```python
from build123d import *

# Parameters (mm, degrees)
SKETCH1_R           = 6.011
SKETCH1_W           = 6.016
SKETCH1_H           = 6.016
BOSS_EXTRUDE1_DEPTH = 5.5
BOSS_EXTRUDE2_START = 2
SKETCH1_3_R         = 8
SKETCH1_3_R_2       = 6.011
SKETCH1_3_W         = 6.016
SKETCH1_3_H         = 6.016
BOSS_EXTRUDE2_DEPTH = 2
FILLET1_R           = 0.5
CUT_EXTRUDE1_DEPTH  = 0.5


with BuildPart() as part:
    # Sketch1 → Boss-Extrude1 (new body)
    with BuildSketch(Plane.XY):
        Circle(SKETCH1_R)
        Rectangle(SKETCH1_W, SKETCH1_H, mode=Mode.SUBTRACT)
    extrude(amount=-BOSS_EXTRUDE1_DEPTH)

    # Sketch1_3 → Boss-Extrude2 (add)
    # profile 1 of 2: a face of its own
    with BuildSketch(Plane.XY.offset(BOSS_EXTRUDE2_START)):
        Circle(SKETCH1_3_R)
        Circle(SKETCH1_3_R_2, mode=Mode.SUBTRACT)
    # profile 2 of 2: a face of its own
    with BuildSketch(Plane.XY.offset(BOSS_EXTRUDE2_START)):
        Circle(SKETCH1_3_R_2)
        Rectangle(SKETCH1_3_W, SKETCH1_3_H, mode=Mode.SUBTRACT)
    extrude(amount=-BOSS_EXTRUDE2_DEPTH)

    # Fillet1
    fillet1_edges = [part.edges().sort_by_distance(p)[0] for p in [
        (-8, 0, 0),
        (-6.011, 0, -5.5),
    ]]
    fillet(fillet1_edges, radius=FILLET1_R)

    # Sketch2 → Cut-Extrude1 (cut)
    with BuildSketch(Plane.XY.offset(2)):
        with BuildLine():
            Line((-0.770976701, 6.337168177), (-1.085079266, 6.337168177))
            add(Edge.make_bspline(
                [(-1.085079266, 6.337168177), (-1.076569715, 6.372400661), (-1.059934239, 6.441277286), (-1.025236666, 6.539684546), (-0.987437411, 6.632808068), (-0.942048306, 6.718904141), (-0.892539552, 6.799703044), (-0.83581683, 6.873372169), (-0.774497108, 6.941785134), (-0.706672158, 7.002498372), (-0.635543497, 7.057476101), (-0.560108877, 7.104351158), (-0.481885983, 7.144675311), (-0.40033285, 7.177895543), (-0.315206679, 7.202921067), (-0.227277055, 7.221077872), (-0.136313555, 7.232868986), (-0.074565965, 7.23401975), (-0.043212278, 7.234604075)],
                knots=[0, 0, 0, 0, 1.162005537, 2.271625781, 3.343758855, 4.383309926, 5.390229558, 6.379919256, 7.361854164, 8.333198761, 9.295911338, 10.242430842, 11.177959212, 12.116337295, 13.062827104, 14.020064771, 14.994644689, 16, 16, 16, 16], degree=3))
            add(Edge.make_bspline(
                [(-0.043212278, 7.234604075), (0.002470464, 7.233224844), (0.092839475, 7.230496469), (0.225602522, 7.205582032), (0.353629341, 7.1661569), (0.475518589, 7.111683173), (0.588737021, 7.04449586), (0.689473208, 6.964531123), (0.776361719, 6.873331821), (0.849256096, 6.772599257), (0.906331095, 6.664943748), (0.948417469, 6.554143591), (0.97403915, 6.440461619), (0.977359707, 6.36370434), (0.979023299, 6.325249107)],
                knots=[0, 0, 0, 0, 1.083050992, 2.142477498, 3.193116406, 4.255571735, 5.30263384, 6.308962982, 7.297363603, 8.282367274, 9.249857812, 10.179914175, 11.08814088, 12, 12, 12, 12], degree=3))
            add(Edge.make_bspline(
                [(0.979023299, 6.325249107), (0.977859708, 6.288242312), (0.97558274, 6.215825757), (0.956249035, 6.11010426), (0.923712772, 6.01046266), (0.878643009, 5.916481498), (0.820301459, 5.828756658), (0.749628762, 5.747090767), (0.6661261, 5.671121609), (0.602847162, 5.627602136), (0.570269292, 5.605197023)],
                knots=[0, 0, 0, 0, 1.024540389, 2.004866551, 2.965041327, 3.920577974, 4.882998113, 5.874504559, 6.905732034, 8, 8, 8, 8], degree=3))
            add(Edge.make_bspline(
                [(0.570269292, 5.605197023), (0.607501047, 5.587218852), (0.681267921, 5.551598894), (0.781818451, 5.481743137), (0.873096326, 5.401086789), (0.924000045, 5.338144136), (0.949576183, 5.306519139)],
                knots=[0, 0, 0, 0, 1.015518401, 2.012035669, 3.001164323, 4, 4, 4, 4], degree=3))
            add(Edge.make_bspline(
                [(0.949576183, 5.306519139), (0.966417526, 5.283461387), (0.999824422, 5.237723471), (1.041059955, 5.164187045), (1.07846907, 5.089835555), (1.107619289, 5.012676149), (1.130193156, 4.933603136), (1.146329188, 4.85248074), (1.156353329, 4.769242717), (1.157788881, 4.712930237), (1.158510478, 4.684624107)],
                knots=[0, 0, 0, 0, 1.025084078, 2.033381695, 3.024893161, 4.013698104, 4.991890475, 5.976764909, 6.982997093, 8, 8, 8, 8], degree=3))
            add(Edge.make_bspline(
                [(1.158510478, 4.684624107), (1.156715965, 4.635614385), (1.153135383, 4.537825584), (1.121131308, 4.393350862), (1.071518068, 4.25212536), (1.001061132, 4.11705052), (0.915193623, 3.990670139), (0.813036299, 3.87759383), (0.69574989, 3.780395226), (0.564944241, 3.699184998), (0.423227113, 3.634267076), (0.271651521, 3.589209633), (0.112401467, 3.559863633), (0.003194169, 3.556716764), (-0.052326862, 3.555116895)],
                knots=[0, 0, 0, 0, 0.955779014, 1.907060117, 2.875433937, 3.871313158, 4.872415639, 5.851225146, 6.836215519, 7.83643374, 8.849228613, 9.86973379, 10.916971861, 12, 12, 12, 12], degree=3))
            add(Edge.make_bspline(
                [(-0.052326862, 3.555116895), (-0.089746162, 3.555985108), (-0.163374867, 3.557693463), (-0.271618365, 3.569372064), (-0.374940065, 3.590702069), (-0.473479663, 3.619405374), (-0.567324699, 3.655797116), (-0.656188804, 3.701115814), (-0.740618698, 3.754427316), (-0.819817649, 3.816360904), (-0.893776217, 3.885642244), (-0.960528941, 3.963501254), (-1.021188734, 4.048498658), (-1.074131372, 4.141621714), (-1.121768325, 4.241666971), (-1.160949282, 4.34991547), (-1.19543485, 4.465399492), (-1.211468315, 4.545877232), (-1.21969465, 4.587168177)],
                knots=[0, 0, 0, 0, 1.048658725, 2.063410685, 3.046034179, 4.001477787, 4.936774919, 5.862367409, 6.792675028, 7.730719943, 8.675894397, 9.627829632, 10.600096036, 11.597688215, 12.626045268, 13.701542398, 14.82072376, 16, 16, 16, 16], degree=3))
            Line((-1.21969465, 4.587168177), (-0.905592086, 4.587168177))
            add(Edge.make_bspline(
                [(-0.905592086, 4.587168177), (-0.897408795, 4.560219164), (-0.881491582, 4.507800992), (-0.854397284, 4.432360687), (-0.823529012, 4.363202633), (-0.790414453, 4.299819511), (-0.755636007, 4.241587109), (-0.716721082, 4.19004524), (-0.676551937, 4.142930038), (-0.646272584, 4.116385426), (-0.631453464, 4.103394139)],
                knots=[0, 0, 0, 0, 1.198163088, 2.33053128, 3.407730985, 4.417276592, 5.372219308, 6.28897303, 7.162600585, 8, 8, 8, 8], degree=3))
            add(Edge.make_bspline(
                [(-0.631453464, 4.103394139), (-0.611856888, 4.088285805), (-0.572724225, 4.058115773), (-0.508955994, 4.019614144), (-0.441891108, 3.986253119), (-0.370076433, 3.960769423), (-0.295061663, 3.939191763), (-0.215634298, 3.925071244), (-0.132495081, 3.915383072), (-0.075727317, 3.914528141), (-0.046717887, 3.914091254)],
                knots=[0, 0, 0, 0, 0.946170439, 1.889420265, 2.845303464, 3.807233317, 4.801018734, 5.828864929, 6.890507805, 8, 8, 8, 8], degree=3))
            add(Edge.make_bspline(
                [(-0.046717887, 3.914091254), (-0.013964385, 3.914707159), (0.050082262, 3.915911509), (0.143537122, 3.926987216), (0.232444569, 3.943117629), (0.315817495, 3.968030612), (0.394748002, 3.998811463), (0.468129652, 4.037459869), (0.536925758, 4.082804591), (0.600255164, 4.134343749), (0.657200671, 4.190765244), (0.707340184, 4.249778315), (0.749964846, 4.311134145), (0.784348424, 4.375172266), (0.811498974, 4.441627495), (0.829982175, 4.510686324), (0.84283369, 4.58178359), (0.843880302, 4.630112559), (0.844407914, 4.654475869)],
                knots=[0, 0, 0, 0, 1.217147791, 2.380027433, 3.494444702, 4.572153297, 5.609568379, 6.639424714, 7.649109417, 8.668170816, 9.669597737, 10.625200337, 11.543417969, 12.441394052, 13.322311151, 14.205496177, 15.095365482, 16, 16, 16, 16], degree=3))
            add(Edge.make_bspline(
                [(0.844407914, 4.654475869), (0.842877612, 4.687087208), (0.839824624, 4.752147617), (0.816516045, 4.847865191), (0.77817718, 4.940088603), (0.724504669, 5.027244393), (0.65916894, 5.108020295), (0.582804033, 5.180091777), (0.494775805, 5.239561868), (0.413755936, 5.280650525), (0.34199078, 5.3086876), (0.280575395, 5.327362564), (0.211818792, 5.34317622), (0.136552443, 5.357888492), (0.054209226, 5.37040984), (-0.035121212, 5.380851656), (-0.131456973, 5.389206697), (-0.198148139, 5.392937792), (-0.232515163, 5.394860485)],
                knots=[0, 0, 0, 0, 1.07054697, 2.135767047, 3.216561865, 4.33974944, 5.486079747, 6.621378074, 7.775625952, 8.963672916, 9.598146892, 10.304877434, 11.070270905, 11.915000392, 12.823868403, 13.805723172, 14.86925407, 16, 16, 16, 16], degree=3))
            Line((-0.232515163, 5.394860485), (-0.232515163, 5.753834844))
            add(Edge.make_bspline(
                [(-0.232515163, 5.753834844), (-0.189213997, 5.754569648), (-0.104397651, 5.756008948), (0.019496654, 5.773416958), (0.137969966, 5.797497586), (0.248396708, 5.834382778), (0.349045422, 5.877223075), (0.436365024, 5.927075285), (0.509132171, 5.982490034), (0.566993242, 6.044322643), (0.610522471, 6.110637691), (0.642349268, 6.179754348), (0.661149595, 6.252278409), (0.663659262, 6.301773077), (0.664920734, 6.32665135)],
                knots=[0, 0, 0, 0, 1.321986639, 2.589447074, 3.816329219, 5.01088745, 6.139805852, 7.153945165, 8.075214402, 8.924034688, 9.728124013, 10.488707548, 11.240355623, 12, 12, 12, 12], degree=3))
            add(Edge.make_bspline(
                [(0.664920734, 6.32665135), (0.664506324, 6.344929095), (0.663681873, 6.381291802), (0.653284595, 6.434416871), (0.637660554, 6.485917817), (0.616180824, 6.535575627), (0.587430626, 6.583045901), (0.553024639, 6.62873335), (0.512056539, 6.672377129), (0.465111092, 6.713057449), (0.414699287, 6.751826686), (0.359449512, 6.784740323), (0.301027637, 6.812885385), (0.239368982, 6.836094887), (0.174273452, 6.853554175), (0.106046894, 6.866090017), (0.034559211, 6.873927671), (-0.014212521, 6.875056087), (-0.039005548, 6.875629716)],
                knots=[0, 0, 0, 0, 0.884392785, 1.759457502, 2.611959086, 3.489218968, 4.37281399, 5.2945488, 6.255912374, 7.266815255, 8.301784654, 9.332968512, 10.37626691, 11.440494194, 12.520033166, 13.637162961, 14.798855837, 16, 16, 16, 16], degree=3))
            add(Edge.make_bspline(
                [(-0.039005548, 6.875629716), (-0.078857216, 6.874238354), (-0.156696792, 6.8715207), (-0.268911709, 6.847717687), (-0.373231043, 6.809739603), (-0.452969709, 6.764406584), (-0.511852284, 6.71965615), (-0.553929222, 6.680573763), (-0.595249732, 6.63714094), (-0.633095409, 6.586682564), (-0.671369386, 6.532615774), (-0.706213947, 6.472192093), (-0.74007364, 6.406987698), (-0.760476189, 6.360892064), (-0.770976701, 6.337168177)],
                knots=[0, 0, 0, 0, 1.472543308, 2.876219568, 4.221790263, 5.565193594, 6.249813518, 6.953379497, 7.687249741, 8.463570142, 9.283606569, 10.136032583, 11.040678096, 12, 12, 12, 12], degree=3))
        make_face()
    extrude(amount=-CUT_EXTRUDE1_DEPTH, mode=Mode.SUBTRACT)


solid = part.part
```
Geometry check sheet. Reference: the model listing, model coordinates, mm. A direction names the side the tool comes from. Coordinates: 2 decimals unless noted, no trailing zeros. Loops run counter-clockwise (first coordinate to the right, second up) from the corner with the lowest first, then second, coordinate; pieces in that order, holes last. Notation, with made-up numbers: (18, 50) - (25, 50) arc R29 cw to (25, 76) - close; hole circle Ø1 at (60, 16). An arc over 180 degrees is marked (long way). One line per item, written item: value. Start each with the question number.
(1) Mould release check, pull along Y, two halves, no side actions. Record for faces 5 (the flat face through (0, 3.008, -2)), 6 (the flat face through (-6, 2, 0)), 7 (the cylindrical face through (-1.73, -7.81, 1.26)): released by +Y, released by -Y, zero draft, split by the parting line, or undercut.
(2) Material ranges on line 1 (X direction, y = 0.25, z = 1.25); line 2 (Z direction, x = 6.25, y = -2.25); line 3 (X direction, y = -0.5, z = -3.75), recorded low to high. Write a range as [from, to].
(3) Cross-section at B-B on z = -3.5. Enter the section's corners in (x, y).
(4) Tool access check on faces 1 (the cylindrical face through (-0.78, 5.96, -2.46)), 2 (the flat face through (0.06, 5.54, 1.5)), 3 (the flat face through (-3.008, 0, -2)), 4 (the flat face through (0, -4, -5.5)). Record the directions out of +Z, -Z, +X, -X, +Y, -Y that give a thin tool (end or side, any length) a straight path to the whole face; none if there is none.
(5) Depth check by flat-ended pin: P1, Ø1.5, axis at y = 1, z = 0, coming from the -X side; P2, Ø3, axis at x = 1, z = -3, coming from the -Y side; P3, Ø1, axis at y = -2, z = -4, coming from the +X side. Enter the tip coordinate at first touch or a pass-through.
(6) Cross-section at A-A on y = 0. Enter the section's corners in (x, z), plus the area to 3 significant figures.
Results below:
1. face 5: undercut
1. face 6: zero draft
1. face 7: split by the parting line
2. line 1: x = [-8, -3.01], [3.01, 8]
2. line 2: z = [0, 2]
2. line 3: x = [-5.99, -3.01], [3.01, 5.99]
3. outline: circle Ø12.02 at (0, 0); hole (-3.01, -3.01) - (3.01, -3.01) - (3.01, 3.01) - (-3.01, 3.01) - close
4. face 1: -Z
4. face 2: +Z
4. face 3: +Z, -Z
4. face 4: -Z, +X, -X, +Y, -Y
5. P1: stops at x = -7.99
5. P2: stops at y = -6.01
5. P3: stops at x = 5.82
6. outline: (-8, 0.5) arc R0.5 ccw to (-7.5, 0) - (-6.01, 0) - (-6.01, -5) arc R0.5 ccw to (-5.51, -5.5) - (-3.01, -5.5) - (-3.01, 2) - (-8, 2) - close; (3.01, -5.5) - (5.51, -5.5) arc R0.5 ccw to (6.01, -5) - (6.01, 0) - (7.5, 0) arc R0.5 ccw to (8, 0.5) - (8, 2) - (3.01, 2) - close
6. area: 52.8 mm2
